For this review, use the dimensioned drawing (mm, ordinates from the lowest corner) and the shaded views. A direction names the side the tool comes from. Give positions to 0.01 mm unless a question says otherwise; leave off trailing zeros. Write each loop counter-clockwise with the first axis right and the second up, starting at its lowest first coordinate (ties: lowest second). Pieces come first, ordered by that corner, then holes. Notation, with made-up numbers: M -28,80 L 15,80 A24 ccw 15,110 Z; hole C -37.75,58 d4. An arc over 180 degrees is marked long. One line per item, written item: value. Start each with the question number.
Item 1: Consider section D-D, the plane y = 8. Write out the cut boundary in (x, z) (1 decimal).
Item 2: To check wall thickness, follow probe 1 along X at (y, z) = (1.25, 4.25); probe 2 along Y at (x, z) = (9.5, 2.5) (1 decimal); probe 3 along Y at (x, z) = (8.5, 4) (1 decimal). State the ranges of each line that lie inside material, in increasing order.
Item 3: Tool access review of the marked faces 1, 2 and 3: name each direction out of +Z, -Z, +X, -X, +Y, -Y from which nothing blocks a thin tool from reaching the whole face with its end or side.
Item 4: Consider section B-B, the plane x = 6.35. Write out the cut boundary in (y, z) (1 decimal).
Item 5: Clearance check with flat-ended pins moving along their axes: pin 1 Ø0.5 at (x, y) = (3.5, 3.5) entering from +Z; pin 2 Ø0.5 at (x, y) = (6.5, 4) entering from -Z; pin 3 Ø0.8 at (y, z) = (8, 3.5) entering from +X. State where each tip first meets the part, or that it passes through.
Item 6: Consider section A-A, the plane y = 1. Write out the cut boundary in (x, z).
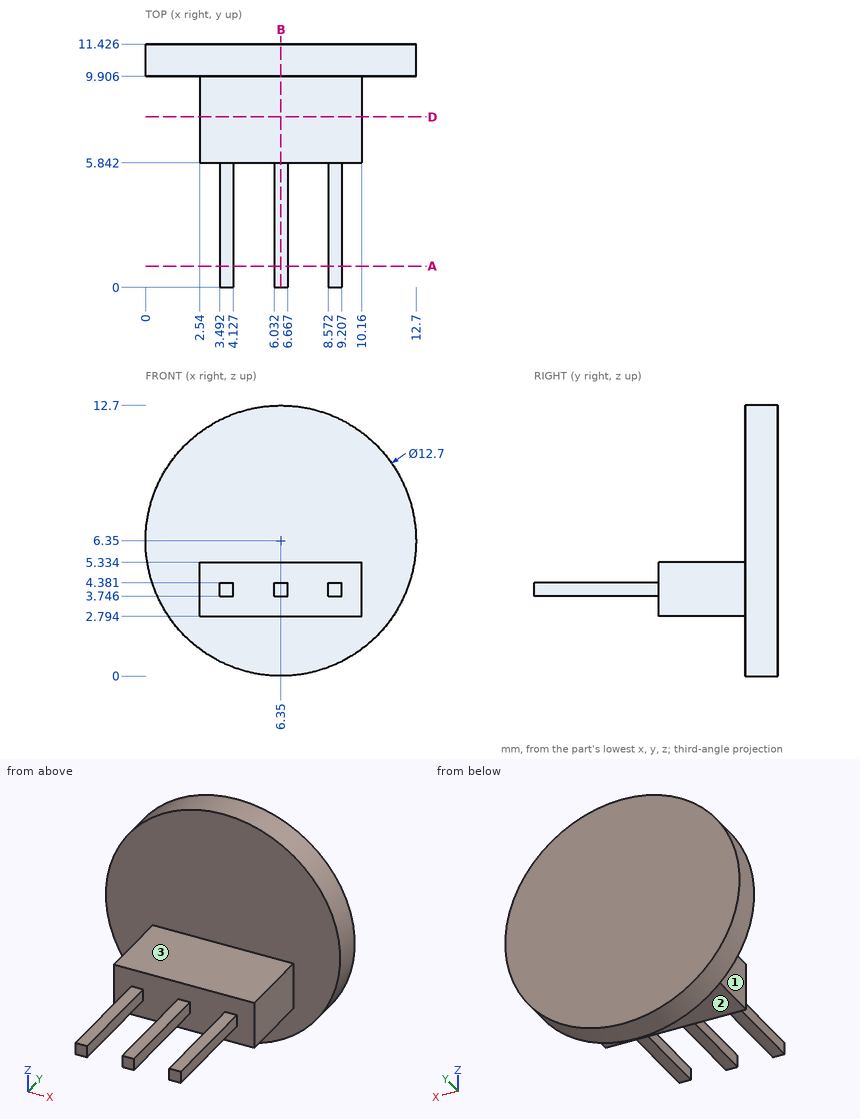
Model answer:
1. outline: M 2.5,2.8 L 10.2,2.8 L 10.2,5.3 L 2.5,5.3 Z
2. probe 1: x = 3.49 to 4.13, 6.03 to 6.67, 8.57 to 9.21
2. probe 2: y = 9.9 to 11.4
2. probe 3: y = 5.8 to 11.4
3. face 1: +Z, -Z, -X, -Y
3. face 2: -Z, +X, -X, -Y
3. face 3: +Z, +X, -X, -Y
4. outline: M 0,3.7 L 5.8,3.7 L 5.8,2.8 L 9.9,2.8 L 9.9,0 L 11.4,0 L 11.4,12.7 L 9.9,12.7 L 9.9,5.3 L 5.8,5.3 L 5.8,4.4 L 0,4.4 Z
5. pin 1: stops at z = 4.38
5. pin 2: stops at z = 3.75
5. pin 3: stops at x = 10.16
6. outline: M 3.49,3.75 L 4.13,3.75 L 4.13,4.38 L 3.49,4.38 Z; M 6.03,3.75 L 6.67,3.75 L 6.67,4.38 L 6.03,4.38 Z; M 8.57,3.75 L 9.21,3.75 L 9.21,4.38 L 8.57,4.38 Z
